```python
from build123d import *

# Parameters (mm, degrees)
BOSS_EXTRUDE1_DEPTH = 15
BOSS_EXTRUDE2_DEPTH = 2
SKETCH3_R           = 1.5
CUT_EXTRUDE1_DEPTH  = 41.669398815
FILLET1_R           = 10
CUT_EXTRUDE4_DEPTH  = 2
FILLET2_R           = 0.5
SKETCH5_W           = 20
SKETCH5_H           = 3
BOSS_EXTRUDE3_DEPTH = 30
SKETCH6_W           = 3
SKETCH6_H           = 3
BOSS_EXTRUDE4_DEPTH = 10
CHAMFER1_SIZE2      = 10
CHAMFER1_SIZE       = 2.679491924
FILLET3_R           = 5
FILLET4_R           = 2


# Some blends are built 0.0001 mm under size
with BuildPart() as part:
    # Sketch1 → Boss-Extrude1 (new, symmetric)
    with BuildSketch(Plane(origin=(0, 0, 0), x_dir=(1, 0, 0), z_dir=(0, 1, 0))):
        Polygon((10, 0), (-10, 0), (-10, 30), (-13, 30), (-13, -3), (-23, -3), (-23, -6), (23, -6), (23, -3), (13, -3), (13, 30), (10, 30), align=None)
    extrude(amount=BOSS_EXTRUDE1_DEPTH, both=True)

    # Sketch2 → Boss-Extrude2 (add, symmetric)
    with BuildSketch(Plane(origin=(0, 0, 0), x_dir=(1, 0, 0), z_dir=(0, 1, 0))):
        Polygon((13, 30), (13, -3), (23, -3), align=None)
    boss_extrude2 = extrude(amount=BOSS_EXTRUDE2_DEPTH, both=True)

    # Mirror1: Boss-Extrude2 across plane
    add(boss_extrude2.mirror(Plane(origin=(0, 0, 0), x_dir=(0, 0, 1), z_dir=(1, 0, 0))))

    # Sketch3 → Cut-Extrude1 (cut, through all)
    with BuildSketch(Plane(origin=(0, 0, 0), x_dir=(-1, 0, 0), z_dir=(0, 0, -1))):
        with Locations((0, -11)):
            Circle(SKETCH3_R)
    extrude(amount=-CUT_EXTRUDE1_DEPTH, mode=Mode.SUBTRACT)

    # Fillet1
    fillet1_edges = [part.edges().sort_by_distance(p)[0] for p in [
        (23, 15, 4.5),
        (-23, 15, 4.5),
    ]]
    fillet(fillet1_edges, radius=FILLET1_R)

    # Sketch4 → Cut-Extrude4 (cut)
    with BuildSketch(Plane(origin=(0, 0, 0), x_dir=(-1, 0, 0), z_dir=(0, 0, -1))):
        with BuildLine():
            Line((0, -15), (4, -15))
            Line((4, -15), (4, -11))
            ThreePointArc((4, -11), (0, -7), (-4, -11))
            Line((-4, -11), (-4, -15))
            Line((-4, -15), (0, -15))
        make_face()
    extrude(amount=-CUT_EXTRUDE4_DEPTH, mode=Mode.SUBTRACT)

    # Fillet2
    fillet2_edges = [part.edges().sort_by_distance(p)[0] for p in [
        (4, -13, 2),
        (0, -7, 2),
        (-4, -13, 2),
    ]]
    fillet(fillet2_edges, radius=FILLET2_R)

    # Sketch5 → Boss-Extrude3 (add)
    with BuildSketch(Plane(origin=(0, 0, 0), x_dir=(-1, 0, 0), z_dir=(0, 0, -1))):
        with Locations((0, 13.5)):
            Rectangle(SKETCH5_W, SKETCH5_H)
    extrude(amount=BOSS_EXTRUDE3_DEPTH)

    # Sketch6 → Boss-Extrude4 (add)
    with BuildSketch(Plane(origin=(23, 0, 0), x_dir=(0, 0, -1), z_dir=(1, 0, 0))):
        with Locations((-4.5, -13.5)):
            Rectangle(SKETCH6_W, SKETCH6_H)
    extrude(amount=BOSS_EXTRUDE4_DEPTH)

    # Chamfer1
    chamfer1_edges = [part.edges().sort_by_distance(p)[0] for p in [
        (23, -12, 4.5),
    ]]
    chamfer1_side = [part.faces().sort_by_distance(p)[0] for p in [
        (23, -11.946410162, 4.5),
    ]]
    chamfer(chamfer1_edges, length=CHAMFER1_SIZE - 0.0001, length2=CHAMFER1_SIZE2 - 0.0001, reference=chamfer1_side[0])  # a hair under: the kernel refuses the full size

    # Fillet3
    fillet3_edges = [part.edges().sort_by_distance(p)[0] for p in [
        (10, 12, -15),
        (0, 12, 0),
        (-10, 12, -15),
        (13, 15, -13.5),
        (-13, 15, -13.5),
    ]]
    fillet(fillet3_edges, radius=FILLET3_R)

    # Fillet4
    # the kernel refuses this fillet: 2 mm, written as the material it adds along each edge
    with BuildSketch(Plane(origin=(-15, 4, 1), x_dir=(0, -1, 0), z_dir=(0, 0, 1))) as fillet4_piece_1_section:
        Polygon((0, 0), (FILLET4_R * 1.02, 0), (FILLET4_R * 1.02, FILLET4_R * 1.02), (0, FILLET4_R * 1.02), align=None)
    fillet4_piece_1 = extrude(amount=FILLET4_R * 1.02, mode=Mode.PRIVATE)
    fillet4_piece_1 = fillet4_piece_1 - Plane(origin=(-15, 4, 1), x_dir=(-0.7071067811865475, 0.7071067811865475, 0), z_dir=(0, 0, 1)) * Sphere(FILLET4_R, mode=Mode.PRIVATE)
    add(fillet4_piece_1)
    with BuildSketch(Plane(origin=(15, 4, 1), x_dir=(-1, 0, 0), z_dir=(0, 0, 1))) as fillet4_piece_2_section:
        Polygon((0, 0), (FILLET4_R * 1.02, 0), (FILLET4_R * 1.02, FILLET4_R * 1.02), (0, FILLET4_R * 1.02), align=None)
    fillet4_piece_2 = extrude(amount=FILLET4_R * 1.02, mode=Mode.PRIVATE)
    fillet4_piece_2 = fillet4_piece_2 - Plane(origin=(15, 4, 1), x_dir=(0.7071067811865475, 0.7071067811865475, 0), z_dir=(0, 0, 1)) * Sphere(FILLET4_R, mode=Mode.PRIVATE)
    add(fillet4_piece_2)
    with BuildSketch(Plane(origin=(15, -4, 1), x_dir=(0, 1, 0), z_dir=(-1, 0, 0))) as fillet4_piece_3_section:
        Polygon((0, 0), (FILLET4_R * 1.02, 0), (FILLET4_R * 1.02, -FILLET4_R * 1.02), (0, -FILLET4_R * 1.02), align=None)
    fillet4_piece_3 = extrude(amount=FILLET4_R * 1.02, mode=Mode.PRIVATE)
    fillet4_piece_3 = fillet4_piece_3 - Plane(origin=(15, -4, 1), x_dir=(0, -0.7071067811865475, -0.7071067811865475), z_dir=(-1, 0, 0)) * Sphere(FILLET4_R, mode=Mode.PRIVATE)
    add(fillet4_piece_3)
    with BuildSketch(Plane(origin=(-15, -4, 1), x_dir=(1, 0, 0), z_dir=(0, 0, 1))) as fillet4_piece_4_section:
        Polygon((0, 0), (FILLET4_R * 1.02, 0), (FILLET4_R * 1.02, FILLET4_R * 1.02), (0, FILLET4_R * 1.02), align=None)
    fillet4_piece_4 = extrude(amount=FILLET4_R * 1.02, mode=Mode.PRIVATE)
    fillet4_piece_4 = fillet4_piece_4 - Plane(origin=(-15, -4, 1), x_dir=(-0.7071067811865475, -0.7071067811865475, 0), z_dir=(0, 0, 1)) * Sphere(FILLET4_R, mode=Mode.PRIVATE)
    add(fillet4_piece_4)
    with BuildSketch(Plane(origin=(23, -9.320608076, 3), x_dir=(0, 1, 0), z_dir=(0, 0, 1))) as fillet4_piece_5:
        with BuildLine():
            CenterArc((FILLET4_R * 0.767332413902, -FILLET4_R), FILLET4_R, 90, 75.000391344)
            Line((-FILLET4_R * 0.19859518016, -FILLET4_R * 0.741187552406), (0, 0))
            Line((0, 0), (FILLET4_R * 0.767332413902, 0))
        make_face()
    extrude(amount=3)
    with BuildSketch(Plane(origin=(-13, 4, 3), x_dir=(-1, 0, 0), z_dir=(0, 1, 0))) as fillet4_piece_6:
        with BuildLine():
            CenterArc((FILLET4_R, -FILLET4_R), FILLET4_R, 90, 90)
            Line((0, -FILLET4_R), (0, 0))
            Line((0, 0), (FILLET4_R, 0))
        make_face()
    extrude(amount=6)
    with BuildSketch(Plane(origin=(13, 4, 3), x_dir=(1, 0, 0), z_dir=(0, 1, 0))) as fillet4_piece_7:
        with BuildLine():
            CenterArc((FILLET4_R, FILLET4_R), FILLET4_R, 180, 90)
            Line((0, FILLET4_R), (0, 0))
            Line((0, 0), (FILLET4_R, 0))
        make_face()
    extrude(amount=6)
    with BuildSketch(Plane(origin=(-8, 10, 3), x_dir=(0.8416879607506225, 0.5399642365263265, 0), z_dir=(0.5399642365263265, -0.8416879607506225, 0))) as fillet4_piece_8_section:
        with BuildLine():
            CenterArc((5 + FILLET4_R, -FILLET4_R), FILLET4_R, 90, 90)
            Line((5 + FILLET4_R, 0), (5, 0))
            Line((5, 0), (5, -FILLET4_R))
        make_face()
    fillet4_piece_8 = revolve(axis=Axis((-8, 10, 3), (0, 0, 1)), revolution_arc=147.318795695, mode=Mode.PRIVATE)
    fillet4_piece_8 = split(fillet4_piece_8, bisect_by=Plane(origin=(-11.613068515, 15, 2.473069622), z_dir=(0, -1, 0)), keep=Keep.TOP, mode=Mode.PRIVATE)
    add(fillet4_piece_8)
    with BuildSketch(Plane(origin=(8, 10, 3), x_dir=(-0.8416879607506222, 0.5399642365263269, 0), z_dir=(-0.5399642365263269, -0.8416879607506222, 0))) as fillet4_piece_9_section:
        with BuildLine():
            CenterArc((5 + FILLET4_R, FILLET4_R), FILLET4_R, 180, 90)
            Line((5, FILLET4_R), (5, 0))
            Line((5, 0), (5 + FILLET4_R, 0))
        make_face()
    fillet4_piece_9 = revolve(axis=Axis((8, 10, 3), (0, 0, -1)), revolution_arc=147.318795695, mode=Mode.PRIVATE)
    fillet4_piece_9 = split(fillet4_piece_9, bisect_by=Plane(origin=(11.613076931, 15, 2.472895292), z_dir=(0, -1, 0)), keep=Keep.TOP, mode=Mode.PRIVATE)
    add(fillet4_piece_9)
    with BuildSketch(Plane(origin=(13, -15, 3), x_dir=(1, 0, 0), z_dir=(0, 1, 0)), Plane(origin=(-13, -15, 3), x_dir=(0, 0, -1), z_dir=(0, 1, 0))) as fillet4_piece_10:
        with BuildLine():
            CenterArc((FILLET4_R, FILLET4_R), FILLET4_R, 180, 90)
            Line((0, FILLET4_R), (0, 0))
            Line((0, 0), (FILLET4_R, 0))
        make_face()
    extrude(amount=11)
    with BuildSketch(Plane(origin=(13, -2, -35), x_dir=(0, -1, 0), z_dir=(0, 0, 1))) as fillet4_piece_11_section:
        with BuildLine():
            CenterArc((FILLET4_R, FILLET4_R), FILLET4_R, 180, 90)
            Line((0, FILLET4_R), (0, 0))
            Line((0, 0), (FILLET4_R, 0))
        make_face()
    fillet4_piece_11 = extrude(amount=36, mode=Mode.PRIVATE)
    fillet4_piece_11 = split(fillet4_piece_11, bisect_by=Plane(origin=(17.53556841, -2.455982706, -15.032624248), z_dir=(-0.9570244044334736, 0, 0.29000739528287095)), keep=Keep.TOP, mode=Mode.PRIVATE)
    add(fillet4_piece_11)
    with BuildSketch(Plane(origin=(15, -2, 3), x_dir=(0, -1, 0), z_dir=(1, 0, 0))) as fillet4_piece_12_section:
        with BuildLine():
            CenterArc((FILLET4_R, FILLET4_R), FILLET4_R, 180, 90)
            Line((0, FILLET4_R), (0, 0))
            Line((0, 0), (FILLET4_R, 0))
        make_face()
    fillet4_piece_12 = extrude(amount=13, mode=Mode.PRIVATE)
    fillet4_piece_12 = split(fillet4_piece_12, bisect_by=Plane(origin=(22.535474122, -2.449923656, 1.467064601), z_dir=(-0.9570244044334736, 0, 0.29000739528287095)), keep=Keep.TOP, mode=Mode.PRIVATE)
    add(fillet4_piece_12)
    with BuildSketch(Plane(origin=(13, 2, -35), x_dir=(0, 1, 0), z_dir=(0, 0, 1))) as fillet4_piece_13_section:
        with BuildLine():
            CenterArc((FILLET4_R, -FILLET4_R), FILLET4_R, 90, 90)
            Line((0, -FILLET4_R), (0, 0))
            Line((0, 0), (FILLET4_R, 0))
        make_face()
    fillet4_piece_13 = extrude(amount=36, mode=Mode.PRIVATE)
    fillet4_piece_13 = split(fillet4_piece_13, bisect_by=Plane(origin=(17.53556841, 2.455982706, -15.032624248), z_dir=(-0.9570244044334736, 0, 0.29000739528287095)), keep=Keep.TOP, mode=Mode.PRIVATE)
    add(fillet4_piece_13)
    with BuildSketch(Plane(origin=(15, 2, 3), x_dir=(0, 1, 0), z_dir=(1, 0, 0))) as fillet4_piece_14_section:
        with BuildLine():
            CenterArc((FILLET4_R, -FILLET4_R), FILLET4_R, 90, 90)
            Line((0, -FILLET4_R), (0, 0))
            Line((0, 0), (FILLET4_R, 0))
        make_face()
    fillet4_piece_14 = extrude(amount=13, mode=Mode.PRIVATE)
    fillet4_piece_14 = split(fillet4_piece_14, bisect_by=Plane(origin=(22.535474122, 2.449923656, 1.467064601), z_dir=(-0.9570244044334736, 0, 0.29000739528287095)), keep=Keep.TOP, mode=Mode.PRIVATE)
    add(fillet4_piece_14)
    with BuildSketch(Plane(origin=(-15, 2, 3), x_dir=(0, 1, 0), z_dir=(-1, 0, 0))) as fillet4_piece_15_section:
        with BuildLine():
            CenterArc((FILLET4_R, FILLET4_R), FILLET4_R, 180, 90)
            Line((0, FILLET4_R), (0, 0))
            Line((0, 0), (FILLET4_R, 0))
        make_face()
    fillet4_piece_15 = extrude(amount=13, mode=Mode.PRIVATE)
    fillet4_piece_15 = split(fillet4_piece_15, bisect_by=Plane(origin=(-22.535474122, 2.449923656, 1.467064601), z_dir=(0.9570244044334736, 0, 0.29000739528287095)), keep=Keep.TOP, mode=Mode.PRIVATE)
    add(fillet4_piece_15)
    with BuildSketch(Plane(origin=(-13, 2, -35), x_dir=(0, 1, 0), z_dir=(0, 0, 1))) as fillet4_piece_16_section:
        with BuildLine():
            CenterArc((FILLET4_R, FILLET4_R), FILLET4_R, 180, 90)
            Line((0, FILLET4_R), (0, 0))
            Line((0, 0), (FILLET4_R, 0))
        make_face()
    fillet4_piece_16 = extrude(amount=36, mode=Mode.PRIVATE)
    fillet4_piece_16 = split(fillet4_piece_16, bisect_by=Plane(origin=(-17.53556841, 2.455982706, -15.032624248), z_dir=(0.9570244044334736, 0, 0.29000739528287095)), keep=Keep.TOP, mode=Mode.PRIVATE)
    add(fillet4_piece_16)
    with BuildSketch(Plane(origin=(-13, -2, -35), x_dir=(0, -1, 0), z_dir=(0, 0, 1))) as fillet4_piece_17_section:
        with BuildLine():
            CenterArc((FILLET4_R, -FILLET4_R), FILLET4_R, 90, 90)
            Line((0, -FILLET4_R), (0, 0))
            Line((0, 0), (FILLET4_R, 0))
        make_face()
    fillet4_piece_17 = extrude(amount=36, mode=Mode.PRIVATE)
    fillet4_piece_17 = split(fillet4_piece_17, bisect_by=Plane(origin=(-17.53556841, -2.455982706, -15.032624248), z_dir=(0.9570244044334736, 0, 0.29000739528287095)), keep=Keep.TOP, mode=Mode.PRIVATE)
    add(fillet4_piece_17)
    with BuildSketch(Plane(origin=(-15, -2, 3), x_dir=(0, -1, 0), z_dir=(-1, 0, 0))) as fillet4_piece_18_section:
        with BuildLine():
            CenterArc((FILLET4_R, -FILLET4_R), FILLET4_R, 90, 90)
            Line((0, -FILLET4_R), (0, 0))
            Line((0, 0), (FILLET4_R, 0))
        make_face()
    fillet4_piece_18 = extrude(amount=13, mode=Mode.PRIVATE)
    fillet4_piece_18 = split(fillet4_piece_18, bisect_by=Plane(origin=(-22.535474122, -2.449923656, 1.467064601), z_dir=(0.9570244044334736, 0, 0.29000739528287095)), keep=Keep.TOP, mode=Mode.PRIVATE)
    add(fillet4_piece_18)


solid = part.part
```
Part model, mm, in its own coordinate system. A direction names the side the tool comes from. Round coordinates to 2 decimals unless told otherwise and drop trailing zeros. Write each loop counter-clockwise with the first axis right and the second up, starting at its lowest first coordinate (ties: lowest second). Pieces come first, ordered by that corner, then holes. Notation, with made-up numbers: (-29, 37.5) -> (21, 37.5) arc R32 cw to (21, 74.5) -> close; hole circle Ø11 at (36, -9.75). An arc over 180 degrees is marked (long way). Return JSON: item names as keys, results as strings. Group by question number.
Q1. Probe L1, parallel to X at y = 11, z = -10; L2, parallel to X at y = -7, z = -6; L3, parallel to Y at x = 17, z = -15.5. List the from-to ranges inside material, lowest first. Write a range as [from, to].
Q2. Saw through at B-B on z = -12.5. Write the cut outline in (x, y).
Q3. Saw through at A-A on x = 0. Write the cut outline in (y, z), plus the area to 3 significant figures.
Q4. Which spindle directions (+Z, -Z, +X, -X, +Y, -Y) get a long thin tool onto all of the face, cutting with end or side? Do faces 4 (the flat face through (0, -4, 0)), 5 (the cylindrical face through (-13.57, -2.6, -14.72)), 6 (the flat face through (17, -2, -6)). Say none if no direction does.
Q5. Pin check, flat tips, straight feed: pin 1 (5.5 mm diameter, centred on x = 1.5, y = -11, fed in from -Z); pin 2 (1.2 mm diameter, centred on y = -13, z = 1, fed in from +X); pin 3 (6 mm diameter, centred on x = -20.5, z = -11, fed in from -Y); pin 4 (10 mm diameter, centred on x = -17, y = 9.5, fed in from -Z). Stop position of each tip, or through.
Q6. Saw through at C-C on z = -19. Write the cut outline in (x, y).
Q7. Mould opens along X. For faces 1 (the cylindrical face through (-19.99, 12.15, 4.52)), 2 (the flat face through (-19, -9, 3)), 3 (the cylindrical face through (9, 10, -15)) say: pulls with the +X half, pulls with the -X half, needs draft (parallel to the pull), parting line crosses it, or undercut.
Answer:
{
 "1": {"L1": "[-12.9, -8], [8, 12.9]", "L2": "[-13, -10], [10, 13]", "L3": "[-2, 2]"},
 "2": {"outline": "(-18.3, -2) -> (-15, -2) arc R2 cw to (-13, -4) -> (-13, -15) -> (-10, -15) -> (-10, 7) arc R5 cw to (-5, 12) -> (5, 12) arc R5 cw to (10, 7) -> (10, -15) -> (13, -15) -> (13, -4) arc R2 cw to (15, -2) -> (18.3, -2) -> (18.3, 2) -> (15, 2) arc R2 cw to (13, 4) -> (13, 10) arc R5 ccw to (8, 15) -> (-8, 15) arc R5 ccw to (-13, 10) -> (-13, 4) arc R2 cw to (-15, 2) -> (-18.3, 2) -> close"},
 "3": {"outline": "(-15, 2) -> (-12.5, 2) -> (-12.5, 6) -> (-15, 6) -> close; (-9.5, 2) -> (-7.5, 2) arc R0.5 cw to (-7, 1.5) -> (-7, 0) -> (7, 0) arc R5 cw to (12, -5) -> (12, -30) -> (15, -30) -> (15, 6) -> (-9.5, 6) -> close", "area": "247 mm2"},
 "4": {"face 4": "-Z, -Y", "face 5": "-Z, -X, -Y", "face 6": "-Z, +X, -Y"},
 "5": {"pin 1": "z = 0", "pin 2": "x = 13.09", "pin 3": "y = -2", "pin 4": "z = -30"},
 "6": {"outline": "(-16.33, -2) -> (-15, -2) arc R2 cw to (-13, -4) -> (-13, -15) -> (-10, -15) -> (-10, 7) arc R5 cw to (-5, 12) -> (5, 12) arc R5 cw to (10, 7) -> (10, -15) -> (13, -15) -> (13, -4) arc R2 cw to (15, -2) -> (16.33, -2) -> (16.33, 2) -> (15, 2) arc R2 cw to (13, 4) -> (13, 10) arc R5 ccw to (8, 15) -> (-8, 15) arc R5 ccw to (-13, 10) -> (-13, 4) arc R2 cw to (-15, 2) -> (-16.33, 2) -> close"},
 "7": {"face 1": "pulls with the -X half", "face 2": "needs draft", "face 3": "undercut"}
}
